Here's how the part is built. I have some questions about the finished solid (model axes, mm). Face numbers are marked on the shaded views. A direction names the side the tool comes from. Round coordinates to 2 decimals unless told otherwise and drop trailing zeros. Write each loop counter-clockwise with the first axis right and the second up, starting at its lowest first coordinate (ties: lowest second). Pieces come first, ordered by that corner, then holes. Notation, with made-up numbers: (23.25, 85) -> (32.25, 85) arc R22 cw to (32.25, 112) -> close; hole circle Ø3 at (53.5, 84.25). An arc over 180 degrees is marked (long way). Answer as CSV lines item,"result".
Autodesk Inventor part; units mm, degrees
ref_plane "Work Plane1" through (-32.5, 0, 32.5) normal (0.7071, 0, 0.7071) x (0, 1, 0)
ref_plane "YZ Plane" through (0, 0, 0) normal (1, 0, 0) x (0, 1, 0)
ref_plane "XZ Plane" through (0, 0, 0) normal (0, 1, 0) x (-1, 0, 0)
sketch "Sketch1" plane through (0, 0, 0) normal (0, 1, 0) x (-1, 0, 0)
  line L0 (-32.5, -32.5) -> (32.5, -32.5)
  line L1 (32.5, -32.5) -> (32.5, 32.5)
  line L2 (32.5, 32.5) -> (-32.5, 32.5)
  line L3 (-32.5, 32.5) -> (-32.5, -32.5)
  line L4 (-32.5, -32.5) -> (32.5, 32.5) construction
  line L5 (32.5, -32.5) -> (-32.5, 32.5) construction
  line L6 (-32.5, 0) -> (0, -32.5)
  point P0 (0, 0)
  dimension "d0" = 65
  dimension "d1" = 65
extrude "Extrusion1" add sketch "Sketch1" along normal blind 30 contours L6 L3 L2 L1 L0
sketch "Sketch2" plane through (32.5, 0, 32.5) normal (1, 0, 0) x (0, 0, -1)
  line L0 (0, 0) -> (32.5, 0)
  line L1 (0, 30) -> (32.5, 30)
  line L2 (0, 0) -> (32.5, 30)
  circle A0 centre (16.25, 15) radius 10.8
  dimension "d5" = 21.6
extrude "Extrusion2" cut sketch "Sketch2" against normal blind 65.75
sketch "Sketch3" plane through (0, 0, -32.5) normal (0, 0, -1) x (-1, 0, 0)
  line L0 (32.5, 0) -> (32.5, 30)
  line L1 (0, 0) -> (32.5, 30)
  circle A0 centre (16.25, 15) radius 10.8
  dimension "d8" = 21.6
extrude "Extrusion3" cut sketch "Sketch3" against normal blind 65.75
sketch "Sketch4" plane through (0, 0, -32.5) normal (0, 0, -1) x (-1, 0, 0)
  circle A0 centre (16.25, 15) radius 10.8
  line L0 (0, 0) -> (32.5, 0)
  line L1 (32.5, 0) -> (32.5, 30)
  line L2 (0, 30) -> (32.5, 30)
  line L3 (0, 0) -> (0, 30)
  point P0 (0, 0)
extrude "Extrusion4" add sketch "Sketch4" along normal blind 20
sketch "Sketch6" plane through (-32.5, 0, 32.5) normal (0, 0, 1) x (1, 0, 0)
  point P0 (32.5, 0)
ref_plane "Work Plane1" through (-32.5, 0, 32.5) normal (0.7071, 0, 0.7071) x (0, 1, 0)
mirror "Mirror1" about plane through (-32.5, 0, 32.5) normal (0.7071, 0, 0.7071) of "Extrusion4"
sketch "Sketch7" plane through (0, 30, 0) normal (0, 1, 0) x (1, 0, 0)
  line L0 (0, 0) -> (10, 0)
  line L1 (10, 0) -> (10, 10)
  line L2 (10, 10) -> (0, 10)
  line L3 (0, 10) -> (0, 0)
  dimension "d20" = 10
  dimension "d21" = 10
extrude "Extrusion7" cut sketch "Sketch7" against normal blind 72
sketch "Sketch8" plane through (0, 30, 0) normal (0, 1, 0) x (1, 0, 0)
  point P0 (0, 0)
sketch "Sketch9" plane through (0, 0, 0) normal (0, -1, 0) x (1, 0, 0)
  line L0 (-32.5, 32.5) -> (52.5, 32.5)
  line L1 (0, 32.5) -> (-32.5, 0)
  line L2 (-32.5, 32.5) -> (-32.5, -52.5)
  line L3 (-16.25, 16.25) -> (-27.05, 27.05)
  line L4 (10, -10) -> (0, -10)
  line L5 (0, -10) -> (0, 0)
  line L6 (0, 0) -> (10, 0)
  line L7 (10, 0) -> (10, -10)
  line L8 (-32.5, 32.5) -> (52.5, 32.5)
  line L9 (-32.5, 32.5) -> (-32.5, -52.5)
  line L10 (0, -52.5) -> (-32.5, -52.5)
  line L11 (0, -32.5) -> (0, -52.5)
  line L12 (32.5, 0) -> (0, -32.5)
  line L13 (32.5, 0) -> (52.5, 0)
  line L14 (52.5, 0) -> (52.5, 32.5)
extrude "Extrusion8" cut sketch "Sketch9" against normal blind 77 contours L0 L1 L2
sketch "Sketch10" plane through (52.5, 0, 0) normal (1, 0, 0) x (0, 0, -1)
  line L0 (-32.5, 0) -> (-32.5, 30)
  line L1 (-32.5, 15) -> (70.7005, 15)
  line L2 (-32.5, 18) -> (63.4302, 18)
  line L3 (63.4302, 18) -> (63.4302, 33.0459)
  line L4 (63.4302, 33.0459) -> (-32.5, 33.0459)
  line L5 (-32.5, 33.0459) -> (-32.5, 18)
  line L6 (-32.5, 12) -> (64.9451, 12)
  line L7 (64.9451, 12) -> (64.9451, -20.31)
  line L8 (64.9451, -20.31) -> (-32.5, -20.31)
  line L9 (-32.5, -20.31) -> (-32.5, 12)
  line L10 (32.5, 0) -> (52.5, 0)
  line L11 (-32.5, 30) -> (52.5, 30)
  line L12 (52.5, 30) -> (52.5, 0)
  line L13 (52.5, 0) -> (-32.5, 0)
  line L14 (-32.5, 0) -> (-32.5, 30)
  point P0 (0, 0)
  point P1 (52.5, 15)
  dimension "d26" = 3
  dimension "d27" = 3
extrude "Extrusion9" cut sketch "Sketch10" against normal blind 103.25 contours L0 L2 L12 L1 | L0 L11 L12 L2
sketch "Sketch11" plane through (52.5, 15, 5.45) normal (0, 1, 0) x (1, 0, 0)
  line L0 (-85, 5.45) -> (-85, 57.95)
  line L1 (-85, 47.95) -> (-90, 47.95)
  circle A0 centre (-90, 47.95) radius 1.5
  circle A1 centre (-90, 47.95) radius 5
  line L2 (-90, 52.95) -> (-85, 52.95)
  line L3 (-85, 52.95) -> (-85, 42.95)
  line L4 (-85, 42.95) -> (-90, 42.95)
  line L5 (-90, 42.95) -> (-90, 52.95)
  line L6 (-52.5, 57.95) -> (-85, 57.95)
  line L7 (-68.75, 57.95) -> (-68.75, 39.1834)
  line L8 (-68.75, -10.8) -> (-79.55, 0)
  line L9 (-68.75, -10.8) -> (-16.5653, 41.3847)
  line L10 (-52.5, 47.95) -> (-47.5, 47.95)
  circle A2 centre (-47.5, 47.95) radius 1.5
  circle A3 centre (-47.5, 47.95) radius 5
  line L11 (-47.5, 52.95) -> (-52.5, 52.95)
  line L12 (-52.5, 52.95) -> (-52.5, 42.95)
  line L13 (-52.5, 42.95) -> (-47.5, 42.95)
  line L14 (-47.5, 42.95) -> (-47.5, 52.95)
  line L15 (-10, -27.05) -> (-10, -32.05)
  circle A4 centre (-10, -32.05) radius 1.5
  circle A5 centre (-10, -32.05) radius 5
  line L16 (-5, -32.05) -> (-5, -27.05)
  line L17 (-5, -27.05) -> (-15, -27.05)
  line L18 (-15, -27.05) -> (-15, -32.05)
  line L19 (-15, -32.05) -> (-5, -32.05)
  line L20 (0, 5.45) -> (0, -27.05)
  line L21 (0, -10.8) -> (-18.7666, -10.8)
  line L22 (-10, 5.45) -> (-10, 10.45)
  circle A6 centre (-10, 10.45) radius 1.5
  circle A7 centre (-10, 10.45) radius 5
  line L23 (-5, 10.45) -> (-5, 5.45)
  line L24 (-5, 5.45) -> (-15, 5.45)
  line L25 (-15, 5.45) -> (-15, 10.45)
  line L26 (-15, 10.45) -> (-5, 10.45)
  point P0 (-52.5, 5.45)
  point P1 (-15, -32.05)
  point P2 (-85, 52.95)
  dimension "d30" = 5
  dimension "d31" = 3
  dimension "d32" = 10
extrude "Extrusion10" add sketch "Sketch11" against normal blind 7.5 contours L4 A1 L0 | A1 L2 L0 | A1 L5 A0 L1 | L1 A0 L5 A1 | A1 L5 A0 | A3 L14 A2 L10 | L12 L11 A3 | L10 A2 L14 A3 | A3 L13 L12 | A3 L14 A2 | A5 L19 A4 L15 | L17 L16 A5 | L15 A4 L19 A5 | A5 L18 L17 | A5 L19 A4 | A7 L26 A6 L22 | L24 L25 A7 | L22 A6 L26 A7 | A7 L23 L24 | A7 L26 A6
sketch "Sketch12" plane through (52.5, 15, 5.45) normal (0, 1, 0) x (1, 0, 0)
  line L0 (0, 0) -> (-57.95, 0)
  line L1 (-57.95, 0) -> (-36.25, 21.7)
  line L2 (-52.5, 37.95) -> (-20, 5.45)
  circle A0 centre (-50.45, 22.95) radius 1.5
  line L3 (-57.95, 0) -> (-57.95, 57.95)
  line L4 (-42.5, 15.45) -> (-52.5, 15.45)
  circle A1 centre (-35, 7.5) radius 1.5
  point P0 (-52.5, 5.45)
  dimension "d35" = 7.5
  dimension "d36" = 7.5
  dimension "d37" = 3
extrude "Extrusion11" cut sketch "Sketch12" against normal blind 19
sketch "Sketch13" plane through (52.5, 7.5, 5.45) normal (0, -1, 0) x (1, 0, 0)
  circle A0 centre (-90, -47.95) radius 1.5
  line L0 (-93.4641, -47.95) -> (-91.7321, -44.95)
  line L1 (-91.7321, -44.95) -> (-88.2679, -44.95)
  line L2 (-88.2679, -44.95) -> (-86.5359, -47.95)
  line L3 (-86.5359, -47.95) -> (-88.2679, -50.95)
  line L4 (-88.2679, -50.95) -> (-91.7321, -50.95)
  line L5 (-91.7321, -50.95) -> (-93.4641, -47.95)
  line L6 (-85, -42.95) -> (-90, -42.95)
  arc A1 (-90, -42.95) -> (-90, -52.95) centre (-90, -47.95) ccw
  line L7 (-90, -52.95) -> (-85, -52.95)
  line L8 (-85, -42.95) -> (-85, -52.95)
  circle A2 centre (-90, -47.95) radius 1.5
  point P0 (-52.5, -5.45)
  dimension "d40" = 6
extrude "Extrusion12" add sketch "Sketch13" along normal blind 3 contours L8 L7 A1 L6
sketch "Sketch14" plane through (52.5, 7.5, 5.45) normal (0, -1, 0) x (1, 0, 0)
  circle A0 centre (-47.5, -47.95) radius 1.5
  line L0 (-50.9641, -47.95) -> (-49.2321, -44.95)
  line L1 (-49.2321, -44.95) -> (-45.7679, -44.95)
  line L2 (-45.7679, -44.95) -> (-44.0359, -47.95)
  line L3 (-44.0359, -47.95) -> (-45.7679, -50.95)
  line L4 (-45.7679, -50.95) -> (-49.2321, -50.95)
  line L5 (-49.2321, -50.95) -> (-50.9641, -47.95)
  line L6 (-47.5, -42.95) -> (-52.5, -42.95)
  line L7 (-52.5, -52.95) -> (-52.5, -42.95)
  line L8 (-52.5, -52.95) -> (-47.5, -52.95)
  arc A1 (-47.5, -52.95) -> (-47.5, -42.95) centre (-47.5, -47.95) ccw
  circle A2 centre (-47.5, -47.95) radius 1.5
  point P0 (-52.5, -5.45)
  dimension "d43" = 6
extrude "Extrusion13" add sketch "Sketch14" along normal blind 3 contours A1 L8 L7 L6
sketch "Sketch15" plane through (0, 0, 0) normal (0, -1, 0) x (1, 0, 0)
  circle A0 centre (2.05, -17.5) radius 1.5
  line L0 (-1.4141, -17.5) -> (0.3179, -14.5)
  line L1 (0.3179, -14.5) -> (3.7821, -14.5)
  line L2 (3.7821, -14.5) -> (5.5141, -17.5)
  line L3 (5.5141, -17.5) -> (3.7821, -20.5)
  line L4 (3.7821, -20.5) -> (0.3179, -20.5)
  line L5 (0.3179, -20.5) -> (-1.4141, -17.5)
  circle A1 centre (17.5, -2.05) radius 1.5
  circle A2 centre (17.5, -2.05) radius 5
  point P0 (0, 0)
  dimension "d46" = 6
  dimension "d47" = 10
extrude "Extrusion14" cut sketch "Sketch15" against normal blind 6 contours A0 | L0 L1 L2 L3 L4 L5 | A1 | A2
sketch "Sketch16" plane through (52.5, 15, 5.45) normal (0, 1, 0) x (1, 0, 0)
  circle A0 centre (-50.45, 22.95) radius 1.5
  circle A1 centre (-35, 7.5) radius 1.5
  circle A2 centre (-50.45, 22.95) radius 1.5
  circle A3 centre (-10, 10.45) radius 1.5
  circle A4 centre (-47.5, 47.95) radius 1.5
  line L0 (-57.95, 0) -> (-57.95, 57.95)
  line L1 (0, 0) -> (-57.95, 0)
  line L2 (0, 5.45) -> (0, 0)
  line L3 (-5, 5.45) -> (0, 5.45)
  line L4 (-5, 5.45) -> (-5, 10.45)
  arc A5 (-5, 10.45) -> (-15, 10.45) centre (-10, 10.45) ccw
  line L5 (-15, 10.45) -> (-15, 5.45)
  line L6 (-20, 5.45) -> (-15, 5.45)
  line L7 (-52.5, 37.95) -> (-20, 5.45)
  line L8 (-52.5, 42.95) -> (-52.5, 37.95)
  line L9 (-52.5, 42.95) -> (-47.5, 42.95)
  arc A6 (-47.5, 42.95) -> (-47.5, 52.95) centre (-47.5, 47.95) ccw
  line L10 (-47.5, 52.95) -> (-52.5, 52.95)
  line L11 (-52.5, 57.95) -> (-52.5, 52.95)
  line L12 (-57.95, 57.95) -> (-52.5, 57.95)
  line L13 (-52.5, 5.45) -> (-42.5, 5.45)
  line L14 (-52.5, 15.45) -> (-52.5, 5.45)
  line L15 (-42.5, 15.45) -> (-52.5, 15.45)
  line L16 (-42.5, 5.45) -> (-42.5, 15.45)
  circle A7 centre (-90, 47.95) radius 1.5
  line L17 (-79.55, 57.95) -> (-79.55, 0)
  line L18 (-85, 57.95) -> (-79.55, 57.95)
  line L19 (-85, 52.95) -> (-85, 57.95)
  line L20 (-85, 52.95) -> (-90, 52.95)
  arc A8 (-90, 52.95) -> (-90, 42.95) centre (-90, 47.95) ccw
  line L21 (-90, 42.95) -> (-85, 42.95)
  line L22 (-85, 5.45) -> (-85, 42.95)
  line L23 (-79.55, 0) -> (-85, 5.45)
  circle A9 centre (-10, -32.05) radius 1.5
  line L24 (-57.95, -21.6) -> (0, -21.6)
  line L25 (-52.5, -27.05) -> (-57.95, -21.6)
  line L26 (-15, -27.05) -> (-52.5, -27.05)
  line L27 (-15, -27.05) -> (-15, -32.05)
  arc A10 (-15, -32.05) -> (-5, -32.05) centre (-10, -32.05) ccw
  line L28 (-5, -32.05) -> (-5, -27.05)
  line L29 (0, -27.05) -> (-5, -27.05)
  line L30 (0, -21.6) -> (0, -27.05)
  circle A11 centre (-52.5, 5.45) radius 98.2361
  point P0 (-52.5, 5.45)
extrude "Extrusion15" cut sketch "Sketch16" against normal blind 1.5 contours A0 | A1 | A3 | A4 | L0 L12 L11 L10 A6 L9 L8 L7 L6 L5 A5 L4 L3 L2 L1 | L14 L15 L16 L13 | A7 | L17 L23 L22 L21 A8 L20 L19 L18 | A9 | L24 L30 L29 L28 A10 L27 L26 L25 | A11
properties part number "Shaft_Connector_Top_Corner"
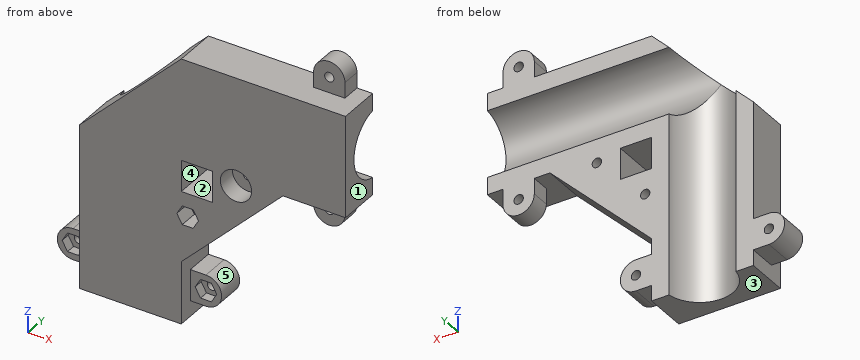
1. For pin 1 Ø4 at (x, y) = (5.5, 2) entering from +Z; pin 2 Ø5 at (x, z) = (17.5, -2.05) entering from -Y; pin 3 Ø3.5 at (x, y) = (-37.5, 6) entering from -Z; pin 4 Ø4 at (x, z) = (-19.5, 18) entering from +Y, each with a flat end and sliding along its axis, tell me the tip position at first contact or that it passes through.
Numbers:
pin 1,"stops at z = 32.5"
pin 2,"stops at y = 6"
pin 3,"stops at z = -47.5"
pin 4,"passes through"
2. Suppose I cut it at B-B on z = -23.5. Please give me the cut outline in (x, y), and give its area (3 significant figures).
Numbers:
outline,"(-32.5, 0) -> (9, 0) -> (9, 13.5) -> (-5.55, 13.5) arc R10.8 cw to (-26.95, 13.5) -> (-32.5, 13.5) -> close"
area,"409 mm^2"
3. Suppose I cut it at C-C on x = 28. Please give me the cut outline in (y, z), and give its area (3 significant figures).
Numbers:
outline,"(0, -4.5) -> (13.5, -4.5) -> (13.5, 5.55) arc R10.8 cw to (13.5, 26.95) -> (13.5, 32.5) -> (0, 32.5) -> close"
area,"349 mm^2"
4. Suppose I cut it at A-A on x = 17.5. Please give me the cut outline in (y, z).
Numbers:
outline,"(0, -15) -> (13.5, -15) -> (13.5, -3.55) -> (6, -3.55) -> (6, -7.05) -> (0, -7.05) -> close; (0, 2.95) -> (6, 2.95) -> (6, -0.55) -> (13.5, -0.55) -> (13.5, 5.55) arc R10.8 cw to (13.5, 26.95) -> (13.5, 32.5) -> (0, 32.5) -> close"
5. If I drill on line 1 (Z direction, x = 2.05, y = 8.75); line 2 (Z direction, x = 5, y = 10.15); line 3 (Z direction, x = 42.5, y = 9.55), over which ranges is the centre line in solid material (lowest first)?
Numbers:
line 1,"z = -47.5 to -37.5, -30.45 to -19, -16 to -10, 0 to 7.44, 25.06 to 32.5"
line 2,"z = -47.5 to -44, -41 to -37.5, -27.5 to -10, 0 to 6.6, 25.9 to 32.5"
line 3,"z = -10 to -6.5, -3.5 to 6.93, 25.57 to 36, 39 to 42.5"
6. Suppose I cut it at D-D on y = 9.75. Count the separate pieces of the cut face and the enclosed holes in it, and give its area (3 significant figures).
Numbers:
separate pieces,"3"
enclosed holes,"7"
area,"2,270 mm^2"
7. On a 3-axis mill with a long thin cutter (end or side, diameter ignored), from which of +Z, -Z, +X, -X, +Y, -Y can I reach the whole of each face in a straight line? I mean the marked faces 4 and 5. Say none if no direction works.
Numbers:
face 4,"+Y, -Y"
face 5,"+X, +Y, -Y"
8. If we mould it in two halves opening along X, with no side actions, what happens to the marked faces 1, 2 and 3? For each: released by +X, released by -X, zero draft, split by the parting line, or undercut.
Numbers:
face 1,"released by +X"
face 2,"undercut"
face 3,"zero draft"
